Could you check a few things on this model? Use its own coordinates, in mm. Face numbers are marked on the shaded views. A direction names the side the tool comes from. Give positions to 0.01 mm unless a question says otherwise; leave off trailing zeros. Write each loop counter-clockwise with the first axis right and the second up, starting at its lowest first coordinate (ties: lowest second). Pieces come first, ordered by that corner, then holes. Notation, with made-up numbers: (-10.75, 34.25) - (-6.75, 34.25) arc R21 cw to (-6.75, 67.25) - close; hole circle Ø8 at (73.5, -38.75). An arc over 180 degrees is marked (long way). Write item = value, one per line.
from build123d import *

# Parameters (mm, degrees)
EXTRUDE_1_DEPTH = 6
EXTRUDE_2_DEPTH = 4.5


with BuildPart() as part:
    # 草图1 → 凸台-拉伸1 (new body)
    with BuildSketch(Plane(origin=(0, 0, 0), x_dir=(1, 0, 0), z_dir=(0, 1, 0))):
        with BuildLine():
            Line((0, 2.85), (3, 2.85))
            ThreePointArc((3, 2.85), (5.85, 0), (3, -2.85))
            Line((3, -2.85), (0, -2.85))
            ThreePointArc((0, -2.85), (-2.85, 0), (0, 2.85))
        make_face()
    extrude(amount=EXTRUDE_1_DEPTH)

    # 草图2 → 凸台-拉伸2 (add)
    with BuildSketch(Plane.XZ):
        with BuildLine():
            Line((0, 4), (3, 4))
            ThreePointArc((3, 4), (7, 0), (3, -4))
            Line((3, -4), (0, -4))
            ThreePointArc((0, -4), (-4, 0), (0, 4))
        make_face()
    extrude(amount=EXTRUDE_2_DEPTH)


solid = part.part
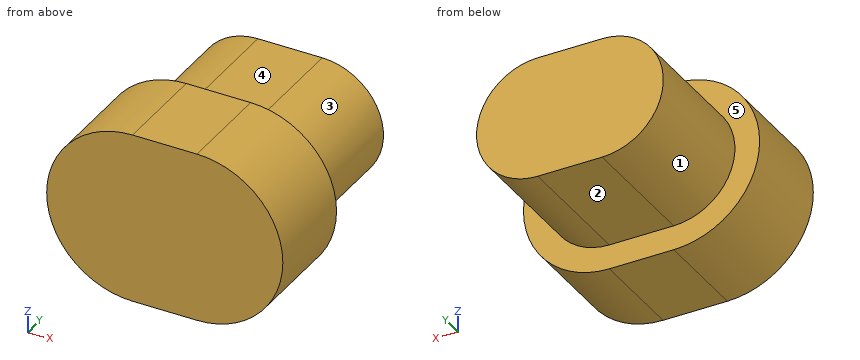
1. For pin 1 (2.5 mm diameter, centred on x = 1.5, y = 2, fed in from +Z); pin 2 (0.9 mm diameter, centred on x = 1.5, y = 3.5, fed in from -Z); pin 3 (3 mm diameter, centred on x = -1.5, y = 3.5, fed in from -Z), each with a flat end and sliding along its axis, tell me the tip position at first contact or that it passes through.
Filled sheet:
pin_1 = 2.85
pin_2 = -2.85
pin_3 = -2.85
2. I need wall thicknesses on line 1 (Y direction, x = 2.75, z = 3.5); line 2 (Z direction, x = 3, y = 1); line 3 (Z direction, x = 4.75, y = -1.25). Which ranges of each line are inside material? Lowest first, please.
Filled sheet:
line_1 = -4.5 to 0
line_2 = -2.85 to 2.85
line_3 = -3.6 to 3.6
3. If we section it at C-C, the plane y = -2.5: Please give me the cut outline in (x, z), and give its area (3 significant figures).
Filled sheet:
outline = (0, -4) - (3, -4) arc R4 ccw to (3, 4) - (0, 4) arc R4 ccw to start
area = 74.3 mm2
4. If we section it at A-A, the plane z = 0: Please give me the cut outline in (x, y).
Filled sheet:
outline = (-4, -4.5) - (7, -4.5) - (7, 0) - (5.85, 0) - (5.85, 6) - (-2.85, 6) - (-2.85, 0) - (-4, 0) - close
5. If we section it at D-D, the plane y = 0.25: Please give me the cut outline in (x, z).
Filled sheet:
outline = (0, -2.85) - (3, -2.85) arc R2.85 ccw to (3, 2.85) - (0, 2.85) arc R2.85 ccw to start
6. Which directions (+Z, -Z, +X, -X, +Y, -Y) give clear straight access to the entire face, cutting with the end or side of a thin tool? Please do the marked faces 1, 2, 3, 4 and 5.
Filled sheet:
face_1 = -X, +Y
face_2 = -Z, +X, -X, +Y
face_3 = +X, +Y
face_4 = +Z, +X, -X, +Y
face_5 = +Y
7. If we section it at B-B, the plane x = 1: Please give me the cut outline in (y, z), and give its area (3 significant figures).
Filled sheet:
outline = (-4.5, -4) - (0, -4) - (0, -2.85) - (6, -2.85) - (6, 2.85) - (0, 2.85) - (0, 4) - (-4.5, 4) - close
area = 70.2 mm2
